Could you check a few things on this drawing? It's one solid part, dimensions in mm from its lowest x, y, z. Give positions to 0.01 mm unless a question says otherwise; leave off trailing zeros. Write each loop counter-clockwise with the first axis right and the second up, starting at its lowest first coordinate (ties: lowest second). Pieces come first, ordered by that corner, then holes. Notation, with made-up numbers: (69, 86.5) -> (82, 86.5) arc R36 ccw to (82, 120.5) -> close; hole circle Ø11 at (2, 68). An arc over 180 degrees is marked (long way). Use CSV: the item, a comma, the result in double quotes. Start each with the question number.
(1) I need wall thicknesses on L1, parallel to Z at x = 6, y = 10.5; L2, parallel to X at y = 9.25, z = 5 (1 decimal); L3, parallel to Z at x = 3.25, y = 12.25. Which ranges of each line are inside material? Lowest first, please. Write a range as [from, to].
(2) If we mould it in two halves opening along Z, with no side actions, what happens to the marked faces 1, 2, 3 and 4? For each: pulls with the +Z half, pulls with the -Z half, needs draft (parallel to the pull), parting line crosses it, or undercut.
(3) Suppose I cut it at A-A on x = 6. List the corners of the cut face in (y, z) for me.
(4) Suppose I cut it at C-C on y = 4.25. List the corners of the cut face in (x, z) for me.
(5) Suppose I cut it at D-D on x = 10.5. List the corners of the cut face in (y, z) for me (1 decimal), plus the area to 3 significant figures.
(6) For pin 1 Ø5 at (x, z) = (6, 5.2) entering from -Y; pin 2 Ø6 at (y, z) = (10.5, 8.5) entering from +X, each with a flat end and sliding along its axis, tell me the tip position at first contact or that it passes through.
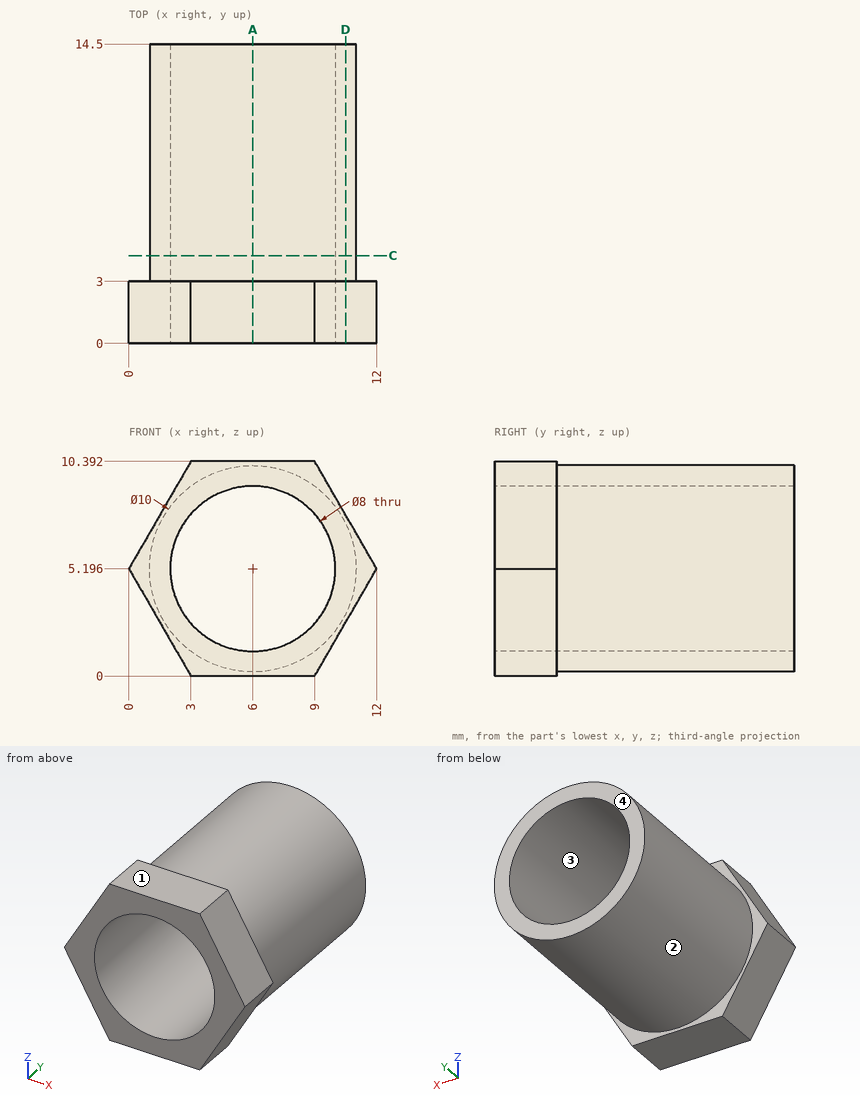
Geometry says:
1,L1,"[0.2, 1.2], [9.2, 10.2]"
1,L2,"[1, 2], [10, 11]"
1,L3,"[1.02, 2.29], [8.1, 9.37]"
2,face 1,"pulls with the +Z half"
2,face 2,"parting line crosses it"
2,face 3,"undercut"
2,face 4,"needs draft"
3,outline,"(0, 0) -> (3, 0) -> (3, 0.2) -> (14.5, 0.2) -> (14.5, 1.2) -> (0, 1.2) -> close; (0, 9.2) -> (14.5, 9.2) -> (14.5, 10.2) -> (3, 10.2) -> (3, 10.39) -> (0, 10.39) -> close"
4,outline,"circle Ø10 at (6, 5.2); hole circle Ø8 at (6, 5.2)"
5,outline,"(0, 2.6) -> (3, 2.6) -> (3, 3) -> (14.5, 3) -> (14.5, 7.4) -> (3, 7.4) -> (3, 7.8) -> (0, 7.8) -> close"
5,area,"65.7 mm²"
6,pin 1,"through"
6,pin 2,"x = 10.99"
